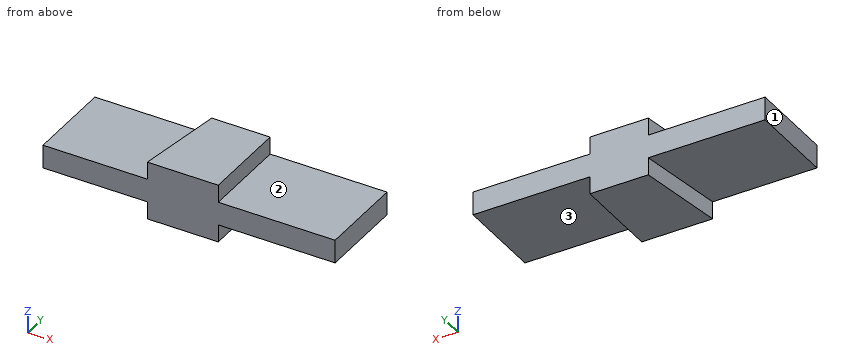
from build123d import *

# Parameters (mm, degrees)
F0_W     = 100
F0_H     = 30
F1_DEPTH = 20
F2_W     = 40
F2_H     = 30
F3_DEPTH = 6
F4_W     = 40
F4_H     = 30
F5_DEPTH = 6


with BuildPart() as f1:
    # F0 (on Top) → F1 (new body)
    with BuildSketch(Plane.XY):
        with Locations((2.482062, -26.390521)):
            Rectangle(F0_W, F0_H)
    extrude(amount=F1_DEPTH)

    # F2 (on face) → F3 (cut)
    with BuildSketch(Plane.XY.offset(20)):
        Polygon((-11.803652, -41.390521), (-7.517938, -11.390521), (-47.517938, -11.390521), (-47.517938, -41.390521), align=None)
        with Locations((32.482062, -26.390521)):
            Rectangle(F2_W, F2_H)
    extrude(amount=-F3_DEPTH, mode=Mode.SUBTRACT)

    # F4 (on face) → F5 (cut)
    with BuildSketch(Plane(origin=(0, 0, 0), x_dir=(1, 0, 0), z_dir=(0, 0, -1))):
        Polygon((-7.517938, 11.390521), (-11.803652, 41.390521), (-47.517938, 41.390521), (-47.517938, 11.390521), align=None)
        with Locations((32.482062, 26.390521)):
            Rectangle(F4_W, F4_H)
    extrude(amount=-F5_DEPTH, mode=Mode.SUBTRACT)


solid = f1.part
Model file for the job. Use its own axes, mm. Face numbers are marked on the shaded views. A direction names the side the tool comes from. Round coordinates to 2 decimals unless told otherwise and drop trailing zeros. Order: outer loops, then holes, each group sorted by start corner. A loop starts at its lowest first (then second) coordinate and runs counter-clockwise, first axis right, second up.
(1) Drill centre lines: line 1 (Z direction, x = -38, y = -38.5); line 2 (X direction, y = -15.25, z = 14.5); line 3 (X direction, y = -35.5, z = 17). Where is each one in solid material? Low to high.
(2) 3-axis set-ups, long thin cutter, end or side, ignore diameter. For the marked faces 1, 2 and 3: which of +Z, -Z, +X, -X, +Y, -Y reach the whole face in a straight line?
(3) Band-saw the part on A-A (y = -24.75). List the corners of the cut face in (x, z), then the cut area to 3 significant figures.
(4) Band-saw the part on B-B (x = 18). List the corners of the cut face in (y, z), then the cut area to 3 significant figures.
(5) Band-saw the part on D-D (y = -14). List the corners of the cut face in (x, z), then the cut area to 3 significant figures.
(6) Pin check, flat tips, straight feed: pin 1 (9 mm diameter, centred on x = -31, y = -26, fed in from -Z); pin 2 (6 mm diameter, centred on x = 18.5, y = -31, fed in from +Z); pin 3 (12 mm diameter, centred on y = -34.5, z = 3, fed in from +X). Stop position of each tip, or through.
(7) Band-saw the part on C-C (z = 16). List the corners of the cut face in (x, y), then the cut area to 3 significant figures.
Verdict:
1. line 1: z = 6 to 14
1. line 2: x = -8.07 to 12.48
1. line 3: x = -10.96 to 12.48
2. face 1: +Z, -Z, -X, +Y, -Y
2. face 2: +Z, +X, +Y, -Y
2. face 3: -Z, +X, +Y, -Y
3. outline: (-47.52, 6) - (-9.43, 6) - (-9.43, 0) - (12.48, 0) - (12.48, 6) - (52.48, 6) - (52.48, 14) - (12.48, 14) - (12.48, 20) - (-9.43, 20) - (-9.43, 14) - (-47.52, 14) - close
3. area: 1,060 mm2
4. outline: (-41.39, 6) - (-11.39, 6) - (-11.39, 14) - (-41.39, 14) - close
4. area: 240 mm2
5. outline: (-47.52, 6) - (-7.89, 6) - (-7.89, 0) - (12.48, 0) - (12.48, 6) - (52.48, 6) - (52.48, 14) - (12.48, 14) - (12.48, 20) - (-7.89, 20) - (-7.89, 14) - (-47.52, 14) - close
5. area: 1,040 mm2
6. pin 1: stops at z = 6
6. pin 2: stops at z = 14
6. pin 3: stops at x = 52.48
7. outline: (-11.8, -41.39) - (12.48, -41.39) - (12.48, -11.39) - (-7.52, -11.39) - close
7. area: 664 mm2
